```python
from build123d import *

# Parameters (mm, degrees)
BASPROSKE_W         = 15
BASPROSKE_H         = 18
TOOTHCUT_DEPTH      = 30.546573405
TEETHCUTS_COUNT     = 16
TEETHCUTS_ANGLE     = 337.5
HUBNEABOTSKE_R      = 5
HUBNEARBOTH_DEPTH   = 15.0000254
HUBFAR_START        = 15.0000254
HUBFARSKE_R         = 5
HUBFAR_DEPTH        = 15.0000254
BORSKE_R            = 2.5
BORE_DEPTH          = 45.0000508
BOSS_EXTRUDE1_DEPTH = 45.0000508
CUT_EXTRUDE1_DEPTH  = 52.521769281


with BuildPart() as part:
    # BasProSke → Base-Revolve (revolve)
    with BuildSketch(Plane(origin=(0, 0, 0), x_dir=(1, 0, 0), z_dir=(0, 1, 0)), mode=Mode.PRIVATE) as base_revolve_sk:
        with Locations((7.5, 9)):
            Rectangle(BASPROSKE_W, BASPROSKE_H)
    revolve(base_revolve_sk.sketch.rotate(Axis((-10, 0, 0), (1, 0, 0)), 180), axis=Axis((-10, 0, 0), (1, 0, 0)))

    # TooCutSke → ToothCut (cut, through all)
    with BuildSketch(Plane(origin=(0, 0, 0), x_dir=(0, 0, -1), z_dir=(1, 0, 0))):
        with BuildLine():
            ThreePointArc((1.03434411, 13.459313997), (0, 13.499), (-1.03434411, 13.459313997))
            ThreePointArc((-1.03434411, 13.459313997), (-1.635143665, 15.806872195), (-3.065655864, 17.762792553))
            ThreePointArc((-3.065655864, 17.762792553), (0, 18.0254), (3.065655864, 17.762792553))
            ThreePointArc((3.065655864, 17.762792553), (1.635143665, 15.806872195), (1.03434411, 13.459313997))
        make_face()
    toothcut = extrude(amount=TOOTHCUT_DEPTH, mode=Mode.SUBTRACT)

    # TeethCuts: ToothCut ×16 about axis
    teethcuts_axis = Axis((-10, 0, 0), (1, 0, 0))
    for i in range(1, TEETHCUTS_COUNT):
        add(toothcut.rotate(teethcuts_axis, i * TEETHCUTS_ANGLE / (TEETHCUTS_COUNT - 1)), mode=Mode.SUBTRACT)

    # HubNeaBotSke → HubNearBoth (add)
    with BuildSketch(Plane.ZY):
        with Locations(Location((0, 0, 0), (0, 0, 180))):
            Circle(HUBNEABOTSKE_R)
    extrude(amount=HUBNEARBOTH_DEPTH)

    # HubFarSke → HubFar (add)
    with BuildSketch(Plane(origin=(15, 0, 0), x_dir=(0, 0, -1), z_dir=(1, 0, 0)).offset(HUBFAR_START)):
        Circle(HUBFARSKE_R)
    extrude(amount=-HUBFAR_DEPTH)

    # BorSke → Bore (cut, symmetric)
    with BuildSketch(Plane(origin=(0, 0, 0), x_dir=(0, 0, -1), z_dir=(1, 0, 0))):
        with Locations(Location((0, 0, 0), (0, 0, 180))):
            Circle(BORSKE_R)
    extrude(amount=BORE_DEPTH, both=True, mode=Mode.SUBTRACT)

    # Sketch1 → Boss-Extrude1 (add)
    with BuildSketch(Plane(origin=(30.0000254, 0, 0), x_dir=(0, 0, -1), z_dir=(1, 0, 0))):
        with BuildLine():
            Line((-1.5, 2), (1.5, 2))
            ThreePointArc((1.5, 2), (0, 2.5), (-1.5, 2))
        make_face()
    extrude(amount=-BOSS_EXTRUDE1_DEPTH)

    # Sketch2 → Cut-Extrude1 (cut, through all)
    with BuildSketch(Plane(origin=(30.0000254, 0, 0), x_dir=(0, 0, -1), z_dir=(1, 0, 0))):
        with BuildLine():
            Line((-1.549193338, 2.15), (1.549193338, 2.15))
            ThreePointArc((1.549193338, 2.15), (0, -2.65), (-1.549193338, 2.15))
        make_face()
        with BuildLine():
            Line((-1.5, 2), (1.5, 2))
            ThreePointArc((1.5, 2), (0, -2.5), (-1.5, 2))
        make_face(mode=Mode.SUBTRACT)
    extrude(amount=-CUT_EXTRUDE1_DEPTH, mode=Mode.SUBTRACT)


solid = part.part
```
Can you work these out from the model? Positions are in its coordinate system, mm. A direction names the side the tool comes from. Coordinates: 2 decimals unless noted, no trailing zeros. Loops run counter-clockwise (first coordinate to the right, second up) from the corner with the lowest first, then second, coordinate; pieces in that order, holes last.
Item 1: Please list where these lines run through material, in increasing order: L1, parallel to Z at x = 12, y = 0; L2, parallel to Y at x = 21.5, z = 0; L3, parallel to Y at x = 13, z = -15.
Answers below:
L1: z = -13.5 to -2.65, 2.65 to 13.5
L2: y = -5 to -2.65, 2.15 to 5
L3: y = -9.95 to -9.07, -4.55 to -1.32, 1.32 to 4.55, 9.07 to 9.95
Item 2: Suppose I cut it at A-A (z = 0). Please give me the cut outline in (x, y), then the cut area to 3 significant figures.
Answers below:
outline: (-15, -5) - (0, -5) - (0, -13.5) - (15, -13.5) - (15, -5) - (30, -5) - (30, -2.65) - (-15, -2.65) - close; (-15, 2.15) - (30, 2.15) - (30, 5) - (15, 5) - (15, 13.5) - (0, 13.5) - (0, 5) - (-15, 5) - close
area: 489 mm2
Item 3: I'm going to push flat-ended pins straight in: pin 1 (3 mm diameter, centred on y = -3.5, z = -8, fed in from -X); pin 2 (12 mm diameter, centred on x = 2, y = -9.5, fed in from -Z); pin 3 (3.5 mm diameter, centred on x = -3, z = 0.5, fed in from -Y). Where does each tip first touch, or does it pass through?
Answers below:
pin 1: stops at x = 0
pin 2: stops at z = -17.66
pin 3: stops at y = -5
Item 4: Which directions (+Z, -Z, +X, -X, +Y, -Y) give clear straight access to the entire face, cutting with the end or side of a thin tool? Please do faces 3 (the face through (7.395, -1.614, 15.762)), 4 (the face through (7.395, 12.466, -5.179)), 5 (the face through (7.4, 13.94, 7.52)).
Answers below:
face 3: +Z, +X, -X
face 4: +X, -X
face 5: +X, -X, +Y
Item 5: Suppose I cut it at C-C (x = -3). Please give me the cut outline in (y, z), then the cut area to 3 significant figures.
Answers below:
outline: circle Ø10 at (0, 0); hole (2.15, -1.55) - (2.15, 1.55) arc R2.65 ccw (long way) to start
area: 57.5 mm2
Item 6: If we mould it in two halves opening along Y, with no side actions, what happens to faces 1 (the face through (7.395, 15.762, 1.614)), 2 (the face through (7.82, -2.65, -0.09))? For each: released by +Y, released by -Y, zero draft, split by the parting line, or undercut.
Answers below:
face 1: released by +Y
face 2: undercut
Item 7: Suppose I cut it at D-D (z = 7.5). Please give me the cut outline in (x, y), then the cut area to 3 significant figures.
Answers below:
outline: (0, -13.92) - (15, -13.92) - (15, 13.92) - (0, 13.92) - close
area: 418 mm2
Item 8: Suppose I cut it at B-B (y = 0). Please give me the cut outline in (x, z), then the cut area to 3 significant figures.
Answers below:
outline: (-15, -5) - (0, -5) - (0, -13.5) - (15, -13.5) - (15, -5) - (30, -5) - (30, -2.65) - (-15, -2.65) - close; (-15, 2.65) - (30, 2.65) - (30, 5) - (15, 5) - (15, 13.5) - (0, 13.5) - (0, 5) - (-15, 5) - close
area: 466 mm2
